For this review, take the finished solid that the model builds, in its own axes (mm). A direction names the side the tool comes from. Round coordinates to 2 decimals unless told otherwise and drop trailing zeros. Order: outer loops, then holes, each group sorted by start corner. A loop starts at its lowest first (then second) coordinate and runs counter-clockwise, first axis right, second up. Notation, with made-up numbers: (11.5, -37.5) - (33.5, -37.5) arc R32 ccw to (33.5, -2.5) - close; hole circle Ø3 at (22, 58.25). An arc over 180 degrees is marked (long way). One line per question, with ' | ' between items.
```python
from build123d import *

# Parameters (mm, degrees)
F0_R          = 22
F0_R_2        = 20
F1_DEPTH      = 100
F1_DEPTH_BACK = 2
F0_R_3        = 24
F2_DEPTH      = 2
F3_START      = 2
F3_DEPTH      = 2
F4_START      = 43
F4_DEPTH      = 2
F5_START      = 47
F5_DEPTH      = 2


with BuildPart() as f1:
    # F0 (on Top) → F1 (new body, two sides)
    with BuildSketch(Plane.XY) as f1_sk:
        Circle(F0_R)
        Circle(F0_R_2, mode=Mode.SUBTRACT)
    extrude(amount=F1_DEPTH)
    extrude(f1_sk.sketch, amount=-F1_DEPTH_BACK)

    # F0 (on Top) → F2 (join)
    with BuildSketch(Plane.XY):
        Circle(F0_R_3)
        Circle(F0_R, mode=Mode.SUBTRACT)
    extrude(amount=-F2_DEPTH)

    # F0 (on Top) → F3 (join)
    with BuildSketch(Plane.XY.offset(F3_START)):
        Circle(F0_R_3)
        Circle(F0_R, mode=Mode.SUBTRACT)
    extrude(amount=F3_DEPTH)

    # F0 (on Top) → F4 (join)
    with BuildSketch(Plane.XY.offset(F4_START)):
        Circle(F0_R_3)
        Circle(F0_R, mode=Mode.SUBTRACT)
    extrude(amount=F4_DEPTH)

    # F0 (on Top) → F5 (join)
    with BuildSketch(Plane.XY.offset(F5_START)):
        Circle(F0_R_3)
        Circle(F0_R, mode=Mode.SUBTRACT)
    extrude(amount=F5_DEPTH)


solid = f1.part
```
(1) We need section A-A on z = 30.5. State the section outline as (x, y) points.
Output values:
outline: circle Ø44 at (0, 0); hole circle Ø40 at (0, 0)
(2) For probe 1 along Z at (x, y) = (21, -11); probe 2 along Y at (x, z) = (0, 57); probe 3 along Y at (x, z) = (0, -0.8), list the stretches that pass through material, from the lowest coordinate up. Write a range as [from, to].
Output values:
probe 1: [-2, 0], [2, 4], [43, 45], [47, 49] | probe 2: [-22, -20], [20, 22] | probe 3: [-24, -20], [20, 24]
(3) For faces 4 (the flat face through (7, -21.2, 43)), 5 (the cylindrical face through (-23.977, 1.055, 2.986)), list the 3-axis set-ups (+Z, -Z, +X, -X, +Y, -Y) from which the entire face can be reached by the end or side of a thin tool; tool diameter is ignored.
Output values:
face 4: none | face 5: +Z, -Z
(4) Insertion check: pin 1 (6 mm diameter, centred on x = 3.5, z = 88.5, fed in from -Y); pin 2 (2 mm diameter, centred on x = -14.5, z = 60, fed in from -Y); pin 3 (14.5 mm diameter, centred on x = -8.5, y = 0, fed in from +Z); pin 4 (8 mm diameter, centred on y = -4, z = 66.5, fed in from -X). Each pin has a flat end and moves straight along its axis. Give the tip position at first contact, or say it passes through.
Output values:
pin 1: y = -21.99 | pin 2: y = -17.37 | pin 3: through | pin 4: x = -22
(5) Mouldability with a two-part tool opening along Z and no side actions: class faces 1 (the flat face through (7, -21.2, 49)), 2 (the flat face through (7, -21.2, 45)), 3 (the cylindrical face through (-4.769, -21.477, 74.857)) as released by +Z, released by -Z, zero draft, split by the parting line, or undercut.
Output values:
face 1: released by +Z | face 2: undercut | face 3: zero draft
